Can you work these out from the model? Positions are in its coordinate system, mm. A direction names the side the tool comes from. Give positions to 0.01 mm unless a question says otherwise; leave off trailing zeros. Order: outer loops, then holes, each group sorted by start corner. A loop starts at its lowest first (then second) coordinate and runs counter-clockwise, first axis right, second up. Notation, with made-up numbers: (69, 52.5) - (105, 52.5) arc R19 ccw to (105, 63.5) - close; hole circle Ø10 at (-20.75, 10.5). An arc over 180 degrees is marked (long way). Answer as a JSON object with one key per item and string values.
```python
from build123d import *

# Parameters (mm, degrees)
F2_W     = 5
F2_H     = 3
F3_DEPTH = 27.301


# Not quite as in the source:
# - ends of sketch curves that miss each other by under 0.0002 mm in the source are joined


with BuildPart() as f1:
    # F0 (on Right) → F1 (revolve)
    with BuildSketch(Plane.YZ):
        Polygon((2.5, 33.5), (0, 33.5), (0, 28), (2.5, 18), (11.8, 18), (11.8, 8.5), (27.3, 8.5), (27.3, 13), (26.5, 13), (26.5, 33.5), (25.5, 33.5), (21.0595629684, 21.3), (19.940437, 21.3), (15.5, 33.5), (12.5, 33.5), (8.0595629684, 21.3), (6.940437, 21.3), align=None)
    revolve(axis=Axis((0, 13.65, 0), (0, 1, 0)))

    # F2 (on Front) → F3 (cut, through all)
    with BuildSketch(Plane.XZ):
        with Locations((0, 8.5)):
            Rectangle(F2_W, F2_H)
    extrude(amount=-F3_DEPTH, mode=Mode.SUBTRACT)


solid = f1.part
```
Q1. Which directions (+Z, -Z, +X, -X, +Y, -Y) give clear straight access to the entire face, cutting with the end or side of a thin tool? Please do faces 1 (the face through (-8, 11.8, 4)), 2 (the face through (-27, 0, -8)), 3 (the face through (-2.5, 19, 9)), 4 (the face through (-2.7, 27.3, -8.5)), 5 (the face through (6.627, 6.663, 21.044)).
Recorded:
{"face 1": "-Y", "face 2": "+Z, -Z, +X, -X, -Y", "face 3": "+Y, -Y", "face 4": "+Z, -Z, +X, -X, +Y", "face 5": "none"}
Q2. I'm going to push flat-ended pins straight in: pin 1 Ø6 at (x, y) = (3, 5) entering from -Z; pin 2 Ø1 at (x, z) = (7, -18) entering from +Y; pin 3 Ø2 at (y, z) = (12, 20.5) entering from -X. Where does each tip first touch, or does it pass through?
Recorded:
{"pin 1": "stops at z = -33.47", "pin 2": "stops at y = 26.5", "pin 3": "stops at x = -27.14"}
Q3. I need wall thicknesses on L1, parallel to X at y = 20.25, z = 0; L2, parallel to Y at x = 26.5, z = 16; L3, parallel to X at y = 15.25, z = 0. Which ranges of each line are inside material? Lowest first, please.
Recorded:
{"L1": "x = -21.3 to -8.5, 8.5 to 21.3", "L2": "y = 0 to 3.43, 11.57 to 16.43, 24.57 to 26.5", "L3": "x = -33.5 to -8.5, 8.5 to 33.5"}
Q4. If we section it at D-D, the plane x = -29: Count the separate pieces of the cut face and the enclosed holes in it, then the cut area to 3 significant figures.
Recorded:
{"separate pieces": "3", "enclosed holes": "0", "area": "362 mm^2"}
Q5. If we section it at C-C, the plane y = 14: Please give me the cut outline in (x, z).
Recorded:
{"outline": "circle Ø67 at (0, 0); hole (-2.5, 8.12) arc R8.5 ccw (long way) to (2.5, 8.12) - (2.5, 10) - (-2.5, 10) - close"}
Q6. We'd pull the mould along X, two halves only. Please class faces 6 (the face through (5.55, 2.38, 17.63)), 7 (the face through (-14, 26.5, 0)), 8 (the face through (-21.372, 21.275, -4.746)): released by +X, released by -X, zero draft, split by the parting line, or undercut.
Recorded:
{"face 6": "undercut", "face 7": "zero draft", "face 8": "split by the parting line"}
